```python
from build123d import *

# Parameters (mm, degrees)
F0_R          = 3
F1_DEPTH      = 20
F3_DEPTH      = 4
F3_DEPTH_BACK = 4
F6_DEPTH      = 1
F9_DEPTH      = 1
F10_DEPTH     = 20


with BuildPart() as f1:
    # F0 (on Front) → F1 (new body)
    with BuildSketch(Plane.XZ):
        with BuildLine():
            ThreePointArc((-4, 0), (0, -4), (4, 0))
            ThreePointArc((4, 0), (2.8284271247, 2.8284271247), (0, 4))
            ThreePointArc((0, 4), (-2.8284271247, 2.8284271247), (-4, 0))
        make_face()
        Circle(F0_R, mode=Mode.SUBTRACT)
    extrude(amount=F1_DEPTH)

    # F2 (on Right) → F3 (join, two sides)
    with BuildSketch(Plane.YZ) as f3_sk:
        Polygon((-5.7886751346, -9.5621778265), (-2, -3), (-3.1547005384, -3), (-6.6547005384, -9.0621778265), align=None)
        Polygon((-9.6547005384, -9.0621778265), (-6.1547005384, -3), (-7.3094010768, -3), (-10.5207259422, -8.5621778265), align=None)
    extrude(amount=F3_DEPTH)
    extrude(f3_sk.sketch, amount=-F3_DEPTH_BACK)

    # F5 (on offset) → F6 (join)
    with BuildSketch(Plane(origin=(0, -0.2009618943, 0.1160254038), x_dir=(-1, 0, 0), z_dir=(0, 0.8660254038, -0.5))):
        Polygon((4, -5), (4, 0), (2, -5), align=None)
        Polygon((-2, -5), (-4, 0), (-4, -5), align=None)
    extrude(amount=-F6_DEPTH)

    # F8 (on offset) → F9 (join)
    with BuildSketch(Plane(origin=(0, -3.3169872981, 1.9150635095), x_dir=(-1, 0, 0), z_dir=(0, 0.8660254038, -0.5))):
        Polygon((4, -7), (4, -2), (2, -7), align=None)
        Polygon((-4, -7), (-2, -7), (-4, -2), align=None)
    extrude(amount=-F9_DEPTH)

    # F0 (on Front) → F10 (join)
    with BuildSketch(Plane.XZ):
        with BuildLine():
            ThreePointArc((-4, 0), (0, -4), (4, 0))
            ThreePointArc((4, 0), (2.8284271247, 2.8284271247), (0, 4))
            ThreePointArc((0, 4), (-2.8284271247, 2.8284271247), (-4, 0))
        make_face()
        Circle(F0_R, mode=Mode.SUBTRACT)
        with BuildLine():
            ThreePointArc((0, 4), (2.8284271247, 2.8284271247), (4, 0))
            Line((4, 0), (4, 4))
            Line((4, 4), (0, 4))
        make_face()
        with BuildLine():
            ThreePointArc((-4, 0), (-2.8284271247, 2.8284271247), (0, 4))
            Line((0, 4), (-4, 4))
            Line((-4, 4), (-4, 0))
        make_face()
    extrude(amount=F10_DEPTH)


solid = f1.part
```
The listing builds one solid part. Answer for the finished solid, in the listing's coordinates (mm). A direction names the side the tool comes from. Coordinates: 2 decimals unless noted, no trailing zeros. Loops run counter-clockwise (first coordinate to the right, second up) from the corner with the lowest first, then second, coordinate; pieces in that order, holes last. Notation, with made-up numbers: M 45,84.5 L 68,84.5 A18 cw 68,116.5 Z; hole C -8.5,13.5 d2. An arc over 180 degrees is marked long. Answer as a JSON object with one key per item and string values. Group by question number.
Item 1: Each of these flat-tipped pins is pushed along its axis until it touches: P1, Ø4, axis at y = -8, z = -4, coming from the +X side; P2, Ø1.5, axis at x = 3, z = -5, coming from the -Y side. Where does it stop, or does it pass through?
Item 2: Section A-A (y = -9) is taken. Write down the section's boundary in (x, z).
Item 3: Determine the mould class of faces 1 (the face through (2, 0, 3)), 2 (the face through (4, -10, 2)), 3 (the face through (-0.06, -10.09, -8.81)), 4 (the face through (0, -5, -4)) for opening direction Y: +Y half, -Y half, draft (parallel to the pull), parting line (faces both ways), or undercut.
Item 4: Consider L1, parallel to Z at x = 0, y = -2; L2, parallel to Z at x = 0, y = -6.25; L3, parallel to Z at x = 2.5, y = -4.75. Determine where each line is inside the solid, lowest interval first.
Item 5: Section C-C (z = 1.75) is taken. Write down the section's boundary in (x, y).
Item 6: Section B-B (x = -0.5) is taken. Write down the section's boundary in (y, z), and give its area (3 significant figures).
Item 7: Section D-D (y = -15) is taken. Write down the section's boundary in (x, z).
Item 8: Which of the six approach directions +Z, -Z, +X, -X, +Y, -Y give full straight-line access (tool end or side, diameter ignored) to faces 5 (the face through (0, -1, -4)), 6 (the face through (0, -13, -4)), 7 (the face through (0, -10, 4))?
Solved:
{
 "1": {"P1": "stops at x = 4", "P2": "stops at y = -8.9"},
 "2": {"outline": "M -4,-7.93 L 4,-7.93 L 4,-5.93 L -4,-5.93 Z; M -4,0 A4 ccw 4,0 L 4,4 L -4,4 Z; hole C 0,0 d6"},
 "3": {"face 1": "+Y half", "face 2": "draft", "face 3": "-Y half", "face 4": "undercut"},
 "4": {"L1": "z = -4 to -3, 3 to 4", "L2": "z = -9.3 to -8.36, -4 to -3, 3 to 4", "L3": "z = -7.76 to -5.76, -3.12 to -1.66, 1.66 to 4"},
 "5": {"outline": "M -4,-20 L -2.44,-20 L -2.44,0 L -4,0 Z; M 2.44,-20 L 4,-20 L 4,0 L 2.44,0 Z"},
 "6": {"outline": "M -20,-3.97 L -7.87,-3.97 L -10.52,-8.56 L -9.65,-9.06 L -6.71,-3.97 L -3.71,-3.97 L -6.65,-9.06 L -5.79,-9.56 L -2.56,-3.97 L 0,-3.97 L 0,-2.96 L -20,-2.96 Z; M -20,2.96 L 0,2.96 L 0,4 L -20,4 Z", "area": "52.8 mm2"},
 "7": {"outline": "M -4,0 A4 ccw 4,0 L 4,4 L -4,4 Z; hole C 0,0 d6"},
 "8": {"face 5": "-Z, +Y", "face 6": "-Y", "face 7": "+Z, +X, -X, +Y, -Y"}
}
